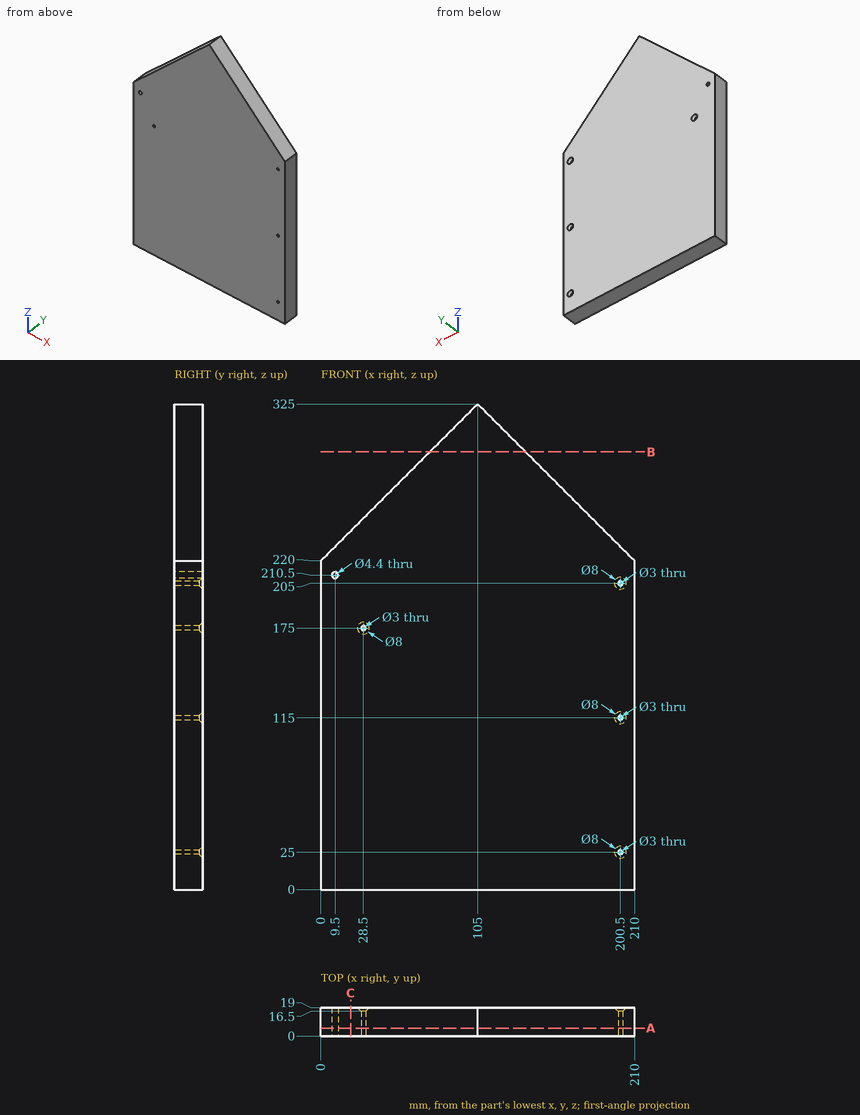
Study the drawing (mm; zero at the part's minimum x, y, z) and answer. Give positions to 0.01 mm unless a question says otherwise; leave off trailing zeros. Write each loop counter-clockwise with the first axis right and the second up, starting at its lowest first coordinate (ties: lowest second). Pieces come first, ordered by that corner, then holes. Notation, with made-up numbers: M 26.5,6.25 L 80.5,6.25 A20 ccw 80.5,32.25 Z; hole C 22.5,2.25 d1. An arc over 180 degrees is marked long. Put each result on its own line as item: value. Start each with the question number.
1. Consider line 1 along X through (y, z) = (5.25, 175); line 2 along Z through (x, y) = (200.5, 6); line 3 along X through (y, z) = (7, 210.5). Determine where each line is inside the solid, lowest interval first.
2. The part is cut by section A-A, the plane y = 5.25. Give the vertices of the cut face in (x, z), and give its area (3 significant figures).
3. The part is cut by section B-B, the plane z = 293. Give the vertices of the cut face in (x, y).
4. The part is cut by section C-C, the plane x = 20. Give the vertices of the cut face in (y, z).
5. Each of these flat-tipped pins is pushed along its axis until it touches: pin 1 Ø5 at (x, z) = (28.5, 175) entering from +Y; pin 2 Ø4 at (x, z) = (200.5, 205) entering from +Y; pin 3 Ø4 at (y, z) = (5.5, 279.5) entering from -X. Where does it stop, or does it pass through?
Final values:
1. line 1: x = 0 to 27, 30 to 210
1. line 2: z = 0 to 23.5, 26.5 to 113.5, 116.5 to 203.5, 206.5 to 229.5
1. line 3: x = 0 to 7.3, 11.7 to 210
2. outline: M 0,0 L 210,0 L 210,220 L 105,325 L 0,220 Z; hole C 9.5,210.5 d4.4; hole C 28.5,175 d3; hole C 200.5,25 d3; hole C 200.5,115 d3; hole C 200.5,205 d3
2. area: 57,200 mm²
3. outline: M 73,0 L 137,0 L 137,19 L 73,19 Z
4. outline: M 0,0 L 19,0 L 19,240 L 0,240 Z
5. pin 1: stops at y = 17.5
5. pin 2: stops at y = 17
5. pin 3: stops at x = 57.5
